```python
from build123d import *

# Parameters (mm, degrees)
BOSS_EXTRUDE1_DEPTH = 5.9
SKETCH2_W           = 8
SKETCH2_H           = 55
BOSS_EXTRUDE2_DEPTH = 5.9
SKETCH3_W           = 9
SKETCH3_H           = 15
SKETCH3_W_2         = 8
SKETCH3_H_2         = 10
CUT_EXTRUDE1_DEPTH  = 6.9
BOSS_EXTRUDE3_DEPTH = 5.9
CUT_EXTRUDE2_REACH  = 7.9
SKETCH5_R           = 2.05


with BuildPart() as part:
    # Sketch1 → Boss-Extrude1 (new body)
    with BuildSketch(Plane.XY):
        with BuildLine():
            ThreePointArc((97.061822228, 90.695765473), (82.799132124, 99.447826237), (76.396720763, 83.987165662))
            Line((76.396720763, 83.987165662), (-17.603279237, 83.987165662))
            Line((-17.603279237, 83.987165662), (-17.603279237, 138.987165662))
            Line((-17.603279237, 138.987165662), (94.396720763, 138.987165662))
            Line((94.396720763, 138.987165662), (94.396720763, 110.289306386))
            ThreePointArc((94.396720763, 110.289306386), (103.949970876, 103.334562845), (108.745956392, 92.534953205))
            Line((108.745956392, 92.534953205), (97.061822228, 90.695765473))
        make_face()
    extrude(amount=BOSS_EXTRUDE1_DEPTH)

    # Sketch2 → Boss-Extrude2 (add)
    with BuildSketch(Plane.XY.offset(5.9)):
        with Locations((-21.603279237, 111.487165662)):
            Rectangle(SKETCH2_W, SKETCH2_H)
    extrude(amount=-BOSS_EXTRUDE2_DEPTH)

    # Sketch3 → Cut-Extrude1 (cut, through all)
    with BuildSketch(Plane.XY.offset(5.9)):
        with Locations((-21.103279237, 111.487165662)):
            Rectangle(SKETCH3_W, SKETCH3_H)
        with Locations((90.396720763, 118.987165662)):
            Rectangle(SKETCH3_W_2, SKETCH3_H_2)
        with Locations((-21.103279237, 88.987165662)):
            Rectangle(SKETCH3_W, SKETCH3_H_2)
    extrude(amount=-CUT_EXTRUDE1_DEPTH, mode=Mode.SUBTRACT)

    # Sketch4 → Boss-Extrude3 (add)
    with BuildSketch(Plane.XY.offset(5.9)):
        Polygon((4.396720763, 138.987165662), (4.396720763, 144.887165662), (-0.603279237, 144.887165662), (-0.603279237, 148.887165662), (19.396720763, 148.887165662), (19.396720763, 144.887165662), (14.396720763, 144.887165662), (14.396720763, 138.987165662), align=None)
        Polygon((49.396720763, 144.887165662), (49.396720763, 148.887165662), (69.396720763, 148.887165662), (69.396720763, 144.887165662), (64.396720763, 144.887165662), (64.396720763, 138.987165662), (54.396720763, 138.987165662), (54.396720763, 144.887165662), align=None)
    extrude(amount=-BOSS_EXTRUDE3_DEPTH)

    # Sketch5 → Cut-Extrude2 (cut, up to next)
    with BuildSketch(Plane.XY.offset(5.9), mode=Mode.PRIVATE) as cut_extrude2_sk1:
        with Locations((-16.603279237, 93.987165662)):
            Circle(SKETCH5_R)
    cut_extrude2_tool1 = extrude(cut_extrude2_sk1.sketch, amount=-CUT_EXTRUDE2_REACH, mode=Mode.PRIVATE) & part.part
    add(cut_extrude2_tool1.solids().sort_by_distance((-16.603279, 93.987166, 5.9))[0], mode=Mode.SUBTRACT)
    # Sketch5 → Cut-Extrude2 (cut, up to next)
    with BuildSketch(Plane.XY.offset(5.9), mode=Mode.PRIVATE) as cut_extrude2_sk2:
        with Locations((-16.603279237, 103.987165662)):
            Circle(SKETCH5_R)
    cut_extrude2_tool2 = extrude(cut_extrude2_sk2.sketch, amount=-CUT_EXTRUDE2_REACH, mode=Mode.PRIVATE) & part.part
    add(cut_extrude2_tool2.solids().sort_by_distance((-16.603279, 103.987166, 5.9))[0], mode=Mode.SUBTRACT)
    # Sketch5 → Cut-Extrude2 (cut, up to next)
    with BuildSketch(Plane.XY.offset(5.9), mode=Mode.PRIVATE) as cut_extrude2_sk3:
        with Locations((-16.603279237, 118.987165662)):
            Circle(SKETCH5_R)
    cut_extrude2_tool3 = extrude(cut_extrude2_sk3.sketch, amount=-CUT_EXTRUDE2_REACH, mode=Mode.PRIVATE) & part.part
    add(cut_extrude2_tool3.solids().sort_by_distance((-16.603279, 118.987166, 5.9))[0], mode=Mode.SUBTRACT)
    # Sketch5 → Cut-Extrude2 (cut, up to next)
    with BuildSketch(Plane.XY.offset(5.9), mode=Mode.PRIVATE) as cut_extrude2_sk4:
        with Locations((4.396720763, 138.987165662)):
            Circle(SKETCH5_R)
    cut_extrude2_tool4 = extrude(cut_extrude2_sk4.sketch, amount=-CUT_EXTRUDE2_REACH, mode=Mode.PRIVATE) & part.part
    add(cut_extrude2_tool4.solids().sort_by_distance((4.396721, 138.987166, 5.9))[0], mode=Mode.SUBTRACT)
    # Sketch5 → Cut-Extrude2 (cut, up to next)
    with BuildSketch(Plane.XY.offset(5.9), mode=Mode.PRIVATE) as cut_extrude2_sk5:
        with Locations((14.396720763, 138.987165662)):
            Circle(SKETCH5_R)
    cut_extrude2_tool5 = extrude(cut_extrude2_sk5.sketch, amount=-CUT_EXTRUDE2_REACH, mode=Mode.PRIVATE) & part.part
    add(cut_extrude2_tool5.solids().sort_by_distance((14.396721, 138.987166, 5.9))[0], mode=Mode.SUBTRACT)
    # Sketch5 → Cut-Extrude2 (cut, up to next)
    with BuildSketch(Plane.XY.offset(5.9), mode=Mode.PRIVATE) as cut_extrude2_sk6:
        with Locations((14.396720763, 144.887165662)):
            Circle(SKETCH5_R)
    cut_extrude2_tool6 = extrude(cut_extrude2_sk6.sketch, amount=-CUT_EXTRUDE2_REACH, mode=Mode.PRIVATE) & part.part
    add(cut_extrude2_tool6.solids().sort_by_distance((14.396721, 144.887166, 5.9))[0], mode=Mode.SUBTRACT)
    # Sketch5 → Cut-Extrude2 (cut, up to next)
    with BuildSketch(Plane.XY.offset(5.9), mode=Mode.PRIVATE) as cut_extrude2_sk7:
        with Locations((4.396720763, 144.887165662)):
            Circle(SKETCH5_R)
    cut_extrude2_tool7 = extrude(cut_extrude2_sk7.sketch, amount=-CUT_EXTRUDE2_REACH, mode=Mode.PRIVATE) & part.part
    add(cut_extrude2_tool7.solids().sort_by_distance((4.396721, 144.887166, 5.9))[0], mode=Mode.SUBTRACT)
    # Sketch5 → Cut-Extrude2 (cut, up to next)
    with BuildSketch(Plane.XY.offset(5.9), mode=Mode.PRIVATE) as cut_extrude2_sk8:
        with Locations((54.396720763, 144.887165662)):
            Circle(SKETCH5_R)
    cut_extrude2_tool8 = extrude(cut_extrude2_sk8.sketch, amount=-CUT_EXTRUDE2_REACH, mode=Mode.PRIVATE) & part.part
    add(cut_extrude2_tool8.solids().sort_by_distance((54.396721, 144.887166, 5.9))[0], mode=Mode.SUBTRACT)
    # Sketch5 → Cut-Extrude2 (cut, up to next)
    with BuildSketch(Plane.XY.offset(5.9), mode=Mode.PRIVATE) as cut_extrude2_sk9:
        with Locations((64.396720763, 144.887165662)):
            Circle(SKETCH5_R)
    cut_extrude2_tool9 = extrude(cut_extrude2_sk9.sketch, amount=-CUT_EXTRUDE2_REACH, mode=Mode.PRIVATE) & part.part
    add(cut_extrude2_tool9.solids().sort_by_distance((64.396721, 144.887166, 5.9))[0], mode=Mode.SUBTRACT)
    # Sketch5 → Cut-Extrude2 (cut, up to next)
    with BuildSketch(Plane.XY.offset(5.9), mode=Mode.PRIVATE) as cut_extrude2_sk10:
        with Locations((64.396720763, 138.987165662)):
            Circle(SKETCH5_R)
    cut_extrude2_tool10 = extrude(cut_extrude2_sk10.sketch, amount=-CUT_EXTRUDE2_REACH, mode=Mode.PRIVATE) & part.part
    add(cut_extrude2_tool10.solids().sort_by_distance((64.396721, 138.987166, 5.9))[0], mode=Mode.SUBTRACT)
    # Sketch5 → Cut-Extrude2 (cut, up to next)
    with BuildSketch(Plane.XY.offset(5.9), mode=Mode.PRIVATE) as cut_extrude2_sk11:
        with Locations((54.396720763, 138.987165662)):
            Circle(SKETCH5_R)
    cut_extrude2_tool11 = extrude(cut_extrude2_sk11.sketch, amount=-CUT_EXTRUDE2_REACH, mode=Mode.PRIVATE) & part.part
    add(cut_extrude2_tool11.solids().sort_by_distance((54.396721, 138.987166, 5.9))[0], mode=Mode.SUBTRACT)
    # Sketch5 → Cut-Extrude2 (cut, up to next)
    with BuildSketch(Plane.XY.offset(5.9), mode=Mode.PRIVATE) as cut_extrude2_sk12:
        with Locations((86.396720763, 123.987165662)):
            Circle(SKETCH5_R)
    cut_extrude2_tool12 = extrude(cut_extrude2_sk12.sketch, amount=-CUT_EXTRUDE2_REACH, mode=Mode.PRIVATE) & part.part
    add(cut_extrude2_tool12.solids().sort_by_distance((86.396721, 123.987166, 5.9))[0], mode=Mode.SUBTRACT)
    # Sketch5 → Cut-Extrude2 (cut, up to next)
    with BuildSketch(Plane.XY.offset(5.9), mode=Mode.PRIVATE) as cut_extrude2_sk13:
        with Locations((86.396720763, 113.987165662)):
            Circle(SKETCH5_R)
    cut_extrude2_tool13 = extrude(cut_extrude2_sk13.sketch, amount=-CUT_EXTRUDE2_REACH, mode=Mode.PRIVATE) & part.part
    add(cut_extrude2_tool13.solids().sort_by_distance((86.396721, 113.987166, 5.9))[0], mode=Mode.SUBTRACT)


solid = part.part
```
Geometry check sheet. Reference: the model listing, model coordinates, mm. A direction names the side the tool comes from. Give positions to 0.01 mm unless a question says otherwise; leave off trailing zeros. Order: outer loops, then holes, each group sorted by start corner. A loop starts at its lowest first (then second) coordinate and runs counter-clockwise, first axis right, second up. Notation, with made-up numbers: (49.5, 63.25) - (97.5, 63.25) arc R7 ccw to (97.5, 72.25) - close; hole circle Ø10 at (21, -32.75). An arc over 180 degrees is marked (long way). Write item = value, one per line. Start each with the question number.
1) Draft check along Y on faces 1 (the cylindrical face through (-15.11, 95.39, 2.99)), 2 (the flat face through (-22, 103.987, 3)), 3 (the flat face through (-22, 93.987, 3)), 4 (the flat face through (41, 117, 5.9)). Enter one of: released by +Y, released by -Y, zero draft, split by the parting line, or undercut.
2) Section check C-C (x = 92). Enter the section's corners in (y, z).
3) Section check A-A (x = 51). Enter the section's corners in (y, z), then the cut area to 3 significant figures.
4) Section check B-B (y = 132). Enter the section's corners in (x, z).
5) Scan lines: L1, parallel to X at y = 95, z = 0.5; L2, parallel to Y at x = 51.5, z = 3.6; L3, parallel to Y at x = 64, z = 2.05. Record each from-to range of solid material in increasing order.
6) Section check D-D (x = 37). Enter the section's corners in (y, z), then the cut area to 4 significant figures.
7) Gauge pin test, flat ends, axial feed: pin 1 Ø1.5 at (y, z) = (106, 5) entering from -X; pin 2 Ø2 at (y, z) = (142, 4) entering from +X; pin 3 Ø3.5 at (x, y) = (-16.6, 93.99) entering from +Z; pin 4 Ø3 at (y, z) = (147, 2.5) entering from -X. Record the tip position at first contact, or that the pin passes through.
8) Access from +Z, -Z, +X, -X, +Y, -Y to the whole of each face (thin tool, end or side, straight path). Record for faces 5 (the flat face through (19.397, 147, 3)), 6 (the flat face through (94.397, 132, 3)), 7 (the flat face through (34, 138.987, 3)).
Geometry check:
q1.face_1 = undercut
q1.face_2 = undercut
q1.face_3 = released by -Y
q1.face_4 = zero draft
q2.outline = (98.33, 0) - (113.99, 0) - (113.99, 5.9) - (98.33, 5.9) - close; (123.99, 0) - (138.99, 0) - (138.99, 5.9) - (123.99, 5.9) - close
q3.outline = (83.99, 0) - (138.99, 0) - (138.99, 5.9) - (83.99, 5.9) - close; (144.89, 0) - (148.89, 0) - (148.89, 5.9) - (144.89, 5.9) - close
q3.area = 348 mm2
q4.outline = (-25.6, 0) - (94.4, 0) - (94.4, 5.9) - (-25.6, 5.9) - close
q5.L1 = -25.6 to -18.39, -14.82 to 76.99, 95.41 to 108.22
q5.L2 = 83.99 to 138.99, 144.89 to 148.89
q5.L3 = 83.99 to 136.98, 141 to 142.88, 146.9 to 148.89
q6.outline = (83.99, 0) - (138.99, 0) - (138.99, 5.9) - (83.99, 5.9) - close
q6.area = 324.5 mm2
q7.pin_1 = -16.6
q7.pin_2 = 64.4
q7.pin_3 = through
q7.pin_4 = -0.6
q8.face_5 = +Z, -Z, +Y
q8.face_6 = +Z, -Z, +X, +Y
q8.face_7 = +Z, -Z
